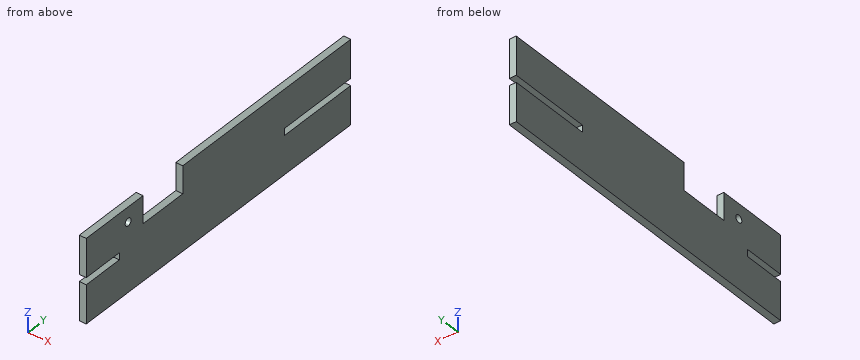
from build123d import *

# Parameters (mm, degrees)
F0_R     = 1.7145
F1_DEPTH = 3.175


with BuildPart() as f1:
    # F0 (on Right) → F1 (new body)
    with BuildSketch(Plane.YZ):
        Polygon((-41.809275, 11.41993), (-74.575491, 11.41993), (-74.575491, -6.04257), (-55.525491, -6.04257), (-55.525491, -7.63007), (39.724509, -7.63007), (39.724509, -6.04257), (58.774509, -6.04257), (77.824509, -6.04257), (77.824509, 11.41993), (-18.942443, 11.41993), (-18.942443, -1.08007), (-41.809275, -1.08007), align=None)
        with Locations((-50.445491, 4.655921)):
            Circle(F0_R, mode=Mode.SUBTRACT)
        Polygon((-55.525491, -9.21757), (-74.575491, -9.21757), (-74.575491, -26.68007), (1.624509, -26.68007), (77.824509, -26.68007), (77.824509, -9.21757), (58.774509, -9.21757), (39.724509, -9.21757), (39.724509, -7.660097), (39.724509, -7.63007), (-55.525491, -7.63007), align=None)
    extrude(amount=F1_DEPTH)


solid = f1.part
Work out the finished part from the listing and answer in its coordinate system (mm). Coordinates: 2 decimals unless noted, no trailing zeros. Order: outer loops, then holes, each group sorted by start corner. A loop starts at its lowest first (then second) coordinate and runs counter-clockwise, first axis right, second up. Notation, with made-up numbers: (79.5, 71.5) - (85.5, 71.5) arc R17 cw to (85.5, 92.5) - close; hole circle Ø7 at (25, 68). An arc over 180 degrees is marked (long way). Put each result on its own line as item: value. Start each with the question number.
1) Find the intervals of material crossed by line 1 (Z direction, x = 3, y = -67.5); line 2 (Y direction, x = 0.8, z = 2.5); line 3 (Z direction, x = 0.7, y = -37.5), in increasing order. Write a range as from..to.
2) Flat-ended cylindrical pins translate along their axes: pin 1 (3 mm diameter, centred on y = -39.5, z = -19, fed in from -X); pin 2 (1 mm diameter, centred on x = 1, z = -8.5, fed in from +Y). Find the tip coordinate at first contact, or state that the pin passes through.
3) Find section B-B (x = 1.25). Give the vertices of the cut face in (y, z).
4) Find section A-A (z = 9.5). Give the vertices of the cut face in (x, y) (1 decimal), plus the area to 3 significant figures.
Results list:
1. line 1: z = -26.68..-9.22, -6.04..11.42
1. line 2: y = -74.58..-41.81, -18.94..77.82
1. line 3: z = -26.68..-1.08
2. pin 1: stops at x = 0
2. pin 2: stops at y = 39.72
3. outline: (-74.58, -26.68) - (77.82, -26.68) - (77.82, -9.22) - (39.72, -9.22) - (39.72, -6.04) - (77.82, -6.04) - (77.82, 11.42) - (-18.94, 11.42) - (-18.94, -1.08) - (-41.81, -1.08) - (-41.81, 11.42) - (-74.58, 11.42) - (-74.58, -6.04) - (-55.53, -6.04) - (-55.53, -9.22) - (-74.58, -9.22) - close; hole circle Ø3.43 at (-50.45, 4.66)
4. outline: (0, -74.6) - (3.2, -74.6) - (3.2, -41.8) - (0, -41.8) - close; (0, -18.9) - (3.2, -18.9) - (3.2, 77.8) - (0, 77.8) - close
4. area: 411 mm^2
